Geometry check sheet. Reference: the model listing, model coordinates, mm. A direction names the side the tool comes from. Round coordinates to 2 decimals unless told otherwise and drop trailing zeros. Loops run counter-clockwise (first coordinate to the right, second up) from the corner with the lowest first, then second, coordinate; pieces in that order, holes last. Notation, with made-up numbers: (-1.75, -18) - (18.25, -18) arc R28 cw to (18.25, 21) - close; hole circle Ø7 at (86, 36.5). An arc over 180 degrees is marked (long way). Write item = value, one per line.
```python
from build123d import *

# Parameters (mm, degrees)
F1_DEPTH = 25.4


with BuildPart() as f1:
    # F0 (on Front) → F1 (new body)
    with BuildSketch(Plane.XZ):
        with BuildLine():
            add(Edge.make_bspline(
                [(-41.275, 9.525), (-40.918331, 65.79854), (12.782067, 63.656478), (54.930287, 62.984836)],
                knots=[0, 0, 0, 0, 110.017253, 110.017253, 110.017253, 110.017253], degree=3))
            Line((-41.275, 9.525), (22.225, 9.525))
            Line((22.225, 9.525), (22.225, 28.130446))
            ThreePointArc((22.225, 28.130446), (31.681597, 52.028481), (54.930287, 62.984836))
        make_face()
        Polygon((22.225, 9.525), (-41.275, 9.525), (-41.275, -9.525), (41.275, -9.525), (41.275, 9.525), align=None)
        with BuildLine():
            Line((22.225, 28.130446), (22.225, 9.525))
            Line((22.225, 9.525), (41.275, 9.525))
            Line((41.275, 9.525), (41.275, 28.130446))
            ThreePointArc((41.275, 28.130446), (47.109768, 40.427169), (60.325, 43.684706))
            Line((60.325, 43.684706), (60.325, 62.910829))
            add(Edge.make_bspline(
                [(54.930287, 62.984836), (56.751848, 62.955809), (58.551832, 62.929529), (60.325, 62.910829)],
                knots=[110.017253, 110.017253, 110.017253, 110.017253, 114.771977, 114.771977, 114.771977, 114.771977], degree=3))
            ThreePointArc((54.930287, 62.984836), (31.681597, 52.028481), (22.225, 28.130446))
        make_face()
        with BuildLine():
            ThreePointArc((60.325, 62.910829), (57.629075, 63.05216), (54.930287, 62.984836))
            add(Edge.make_bspline(
                [(54.930287, 62.984836), (56.751848, 62.955809), (58.551832, 62.929529), (60.325, 62.910829)],
                knots=[110.017253, 110.017253, 110.017253, 110.017253, 114.771977, 114.771977, 114.771977, 114.771977], degree=3))
        make_face()
        Polygon((85.720036, 62.910829), (60.325, 62.910829), (60.325, 43.684706), (60.325, 38.1), (85.687317, 38.1), align=None)
        Polygon((60.325, 66.675), (60.325, 62.910829), (85.720036, 62.910829), (85.725, 66.675), align=None)
        Polygon((85.725, 66.675), (85.720036, 62.910829), (85.687317, 38.1), (111.125, 38.1), (111.125, 66.675), align=None)
    extrude(amount=F1_DEPTH)


solid = f1.part
```
(1) Set-up check for faces 1 (the flat face through (41.275, -13, 9)), 2 (the flat face through (111.125, -13, 52)): record each of +Z, -Z, +X, -X, +Y, -Y from which the full face is reachable in a straight line by a thin tool's end or side.
Answers follow:
face_1 = -Z, +X, +Y, -Y
face_2 = +Z, -Z, +X, +Y, -Y
(2) Gauge pin test, flat ends, axial feed: pin 1 (4.5 mm diameter, centred on y = -16.5, z = 42, fed in from -X); pin 2 (4 mm diameter, centred on x = 80.5, y = -14, fed in from -Z); pin 3 (8 mm diameter, centred on x = 51, y = -13, fed in from -Z). Record the tip position at first contact, or that the pin passes through.
Answers follow:
pin_1 = -33.39
pin_2 = 38.1
pin_3 = 40.34
(3) Section check A-A (x = 63.5). Enter the section's corners in (y, z) (3 decimals).
Answers follow:
outline = (-25.4, 38.1) - (0, 38.1) - (0, 66.675) - (-25.4, 66.675) - close
(4) Scan lines: L1, parallel to X at y = -4, z = 10.5 (3 decimals); L2, parallel to Z at x = 100, y = -1.75 (3 decimals); L3, parallel to Z at x = 27, y = -14.25 (3 decimals). Record each from-to range of solid material in increasing order. Write a range as [from, to].
Answers follow:
L1 = [-41.263, 41.275]
L2 = [38.1, 66.675]
L3 = [-9.525, 63.034]
(5) Mould release check, pull along X, two halves, no side actions. Record for faces 3 (the flat face through (-41.275, -13, 0)), 4 (the flat face through (85, -13, 38.1)), 5 (the cylindrical face through (57.67, -12.52, 63.05)), 6 (the flat face through (60.325, -13, 41)): pulls with the +X half, pulls with the -X half, needs draft (parallel to the pull), parting line crosses it, or undercut.
Answers follow:
face_3 = pulls with the -X half
face_4 = needs draft
face_5 = undercut
face_6 = undercut
